from build123d import *

# Parameters (mm, degrees)
BOSS_EXTRUDE1_DEPTH = 3.175
CUT_EXTRUDE1_REACH  = 5.175
SKETCH2_R           = 2.55


with BuildPart() as part:
    # Model → Boss-Extrude1 (new body)
    with BuildSketch(Plane.XY):
        with BuildLine():
            Line((175, 200), (125, 200))
            ThreePointArc((125, 200), (121.464466094, 198.535533906), (120, 195))
            Line((120, 195), (120, 177.5))
            ThreePointArc((120, 177.5), (118.535533906, 173.964466094), (115, 172.5))
            Line((115, 172.5), (-115, 172.5))
            ThreePointArc((-115, 172.5), (-118.535533906, 173.964466094), (-120, 177.5))
            Line((-120, 177.5), (-120, 195))
            ThreePointArc((-120, 195), (-121.464466094, 198.535533906), (-125, 200))
            Line((-125, 200), (-175, 200))
            ThreePointArc((-175, 200), (-178.535533906, 198.535533906), (-180, 195))
            Line((-180, 195), (-180, -195))
            ThreePointArc((-180, -195), (-178.535533906, -198.535533906), (-175, -200))
            Line((-175, -200), (-125, -200))
            ThreePointArc((-125, -200), (-121.464466094, -198.535533906), (-120, -195))
            Line((-120, -195), (-120, -177.5))
            ThreePointArc((-120, -177.5), (-118.535533906, -173.964466094), (-115, -172.5))
            Line((-115, -172.5), (115, -172.5))
            ThreePointArc((115, -172.5), (118.535533906, -173.964466094), (120, -177.5))
            Line((120, -177.5), (120, -195))
            ThreePointArc((120, -195), (121.464466094, -198.535533906), (125, -200))
            Line((125, -200), (175, -200))
            ThreePointArc((175, -200), (178.535533906, -198.535533906), (180, -195))
            Line((180, -195), (180, 195))
            ThreePointArc((180, 195), (178.535533906, 198.535533906), (175, 200))
        make_face()
    extrude(amount=BOSS_EXTRUDE1_DEPTH)

    # Sketch2 → Cut-Extrude1 (cut, up to next)
    with BuildSketch(Plane.XY.offset(3.175), mode=Mode.PRIVATE) as cut_extrude1_sk1:
        with Locations((-150.5, 190.5)):
            Circle(SKETCH2_R)
    cut_extrude1_tool1 = extrude(cut_extrude1_sk1.sketch, amount=-CUT_EXTRUDE1_REACH, mode=Mode.PRIVATE) & part.part
    add(cut_extrude1_tool1.solids().sort_by_distance((-150.5, 190.5, 3.175))[0], mode=Mode.SUBTRACT)
    # Sketch2 → Cut-Extrude1 (cut, up to next)
    with BuildSketch(Plane.XY.offset(3.175), mode=Mode.PRIVATE) as cut_extrude1_sk2:
        with Locations((-150.5, -190.5)):
            Circle(SKETCH2_R)
    cut_extrude1_tool2 = extrude(cut_extrude1_sk2.sketch, amount=-CUT_EXTRUDE1_REACH, mode=Mode.PRIVATE) & part.part
    add(cut_extrude1_tool2.solids().sort_by_distance((-150.5, -190.5, 3.175))[0], mode=Mode.SUBTRACT)
    # Sketch2 → Cut-Extrude1 (cut, up to next)
    with BuildSketch(Plane.XY.offset(3.175), mode=Mode.PRIVATE) as cut_extrude1_sk3:
        with Locations((150.5, -190.5)):
            Circle(SKETCH2_R)
    cut_extrude1_tool3 = extrude(cut_extrude1_sk3.sketch, amount=-CUT_EXTRUDE1_REACH, mode=Mode.PRIVATE) & part.part
    add(cut_extrude1_tool3.solids().sort_by_distance((150.5, -190.5, 3.175))[0], mode=Mode.SUBTRACT)
    # Sketch2 → Cut-Extrude1 (cut, up to next)
    with BuildSketch(Plane.XY.offset(3.175), mode=Mode.PRIVATE) as cut_extrude1_sk4:
        with Locations((150.5, 190.5)):
            Circle(SKETCH2_R)
    cut_extrude1_tool4 = extrude(cut_extrude1_sk4.sketch, amount=-CUT_EXTRUDE1_REACH, mode=Mode.PRIVATE) & part.part
    add(cut_extrude1_tool4.solids().sort_by_distance((150.5, 190.5, 3.175))[0], mode=Mode.SUBTRACT)


solid = part.part
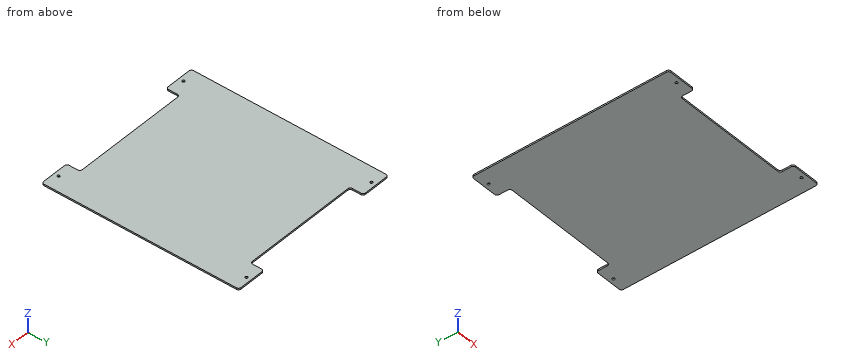
Read the model definition and answer for the solid it produces. Units are mm, in the model's axes. Give positions to 0.01 mm unless a question says otherwise; leave off trailing zeros. Write each loop counter-clockwise with the first axis right and the second up, starting at its lowest first coordinate (ties: lowest second). Pieces come first, ordered by that corner, then holes. Notation, with made-up numbers: M 30,-26.5 L 76,-26.5 A26 cw 76,0.5 Z; hole C 44.25,55.25 d7. An arc over 180 degrees is marked long. One line per item, written item: value. Start each with the question number.
(1) Flat-ended cylindrical pins translate along their axes: pin 1 Ø1.6 at (x, z) = (17.5, 1.5) entering from -Y; pin 2 Ø3 at (x, y) = (-150.5, -190.5) entering from -Z; pin 3 Ø1 at (x, z) = (24.5, 2.5) entering from +Y. Find the tip coordinate at first contact, or state that the pin passes through.
(2) Find section B-B (x = 64). Determine the outline of the cut face in (y, z) (3 decimals).
(3) Find the intervals of material crossed by line 1 (X direction, y = -190.5, z = 2.55); line 2 (Y direction, x = -150.5, z = 2.4); line 3 (Y direction, x = -63, z = 2.05), in increasing order.
(4) Find section A-A (z = 1.6). Determine the outline of the cut face in (x, y).
Results below:
1. pin 1: stops at y = -172.5
1. pin 2: passes through
1. pin 3: stops at y = 172.5
2. outline: M -172.5,0 L 172.5,0 L 172.5,3.175 L -172.5,3.175 Z
3. line 1: x = -180 to -153.05, -147.95 to -120, 120 to 147.95, 153.05 to 180
3. line 2: y = -200 to -193.05, -187.95 to 187.95, 193.05 to 200
3. line 3: y = -172.5 to 172.5
4. outline: M -180,-195 A5 ccw -175,-200 L -125,-200 A5 ccw -120,-195 L -120,-177.5 A5 cw -115,-172.5 L 115,-172.5 A5 cw 120,-177.5 L 120,-195 A5 ccw 125,-200 L 175,-200 A5 ccw 180,-195 L 180,195 A5 ccw 175,200 L 125,200 A5 ccw 120,195 L 120,177.5 A5 cw 115,172.5 L -115,172.5 A5 cw -120,177.5 L -120,195 A5 ccw -125,200 L -175,200 A5 ccw -180,195 Z; hole C -150.5,-190.5 d5.1; hole C -150.5,190.5 d5.1; hole C 150.5,-190.5 d5.1; hole C 150.5,190.5 d5.1
